```python
from build123d import *

# Parameters (mm, degrees)
F1_DEPTH = 20
F2_R     = 18
F3_DEPTH = 30
F6_D     = 10
F7_D     = 14
F7_DEPTH = 31
F7_TIP   = 4.2060243332


with BuildPart() as f1:
    # F0 (on Front) → F1 (new body)
    with BuildSketch(Plane.XZ):
        with BuildLine():
            Line((39.2857142857, 9.0350790291), (10.7142857143, 22.5876975726))
            ThreePointArc((10.7142857143, 22.5876975726), (0, 25), (-10.7142857143, 22.5876975726))
            Line((-10.7142857143, 22.5876975726), (-39.2857142857, 9.0350790291))
            ThreePointArc((-39.2857142857, 9.0350790291), (-45, 0), (-39.2857142857, -9.0350790291))
            Line((-39.2857142857, -9.0350790291), (-10.7142857143, -22.5876975726))
            ThreePointArc((-10.7142857143, -22.5876975726), (0, -25), (10.7142857143, -22.5876975726))
            Line((10.7142857143, -22.5876975726), (39.2857142857, -9.0350790291))
            ThreePointArc((39.2857142857, -9.0350790291), (45, 0), (39.2857142857, 9.0350790291))
        make_face()
    extrude(amount=F1_DEPTH)

    # F2 (on face) → F3 (join)
    with BuildSketch(Plane.XZ.offset(20)):
        Circle(F2_R)
    extrude(amount=F3_DEPTH)

    # F6 (through all)
    with Locations(Plane.XZ.offset(20)):
        with Locations((35, 0), (-35, 0)):
            Hole(F6_D / 2)

    # F7
    with Locations(Plane.XZ.offset(50)):
        with Locations((0, 0)):
            Hole(F7_D / 2, depth=F7_DEPTH)
            with Locations((0, 0, -(F7_DEPTH + F7_TIP / 2))):  # 118° drill point
                Cone(0, F7_D / 2, F7_TIP, mode=Mode.SUBTRACT)


solid = f1.part
```
The listing builds one solid part. Answer for the finished solid, in the listing's coordinates (mm). A direction names the side the tool comes from. Give positions to 0.01 mm unless a question says otherwise; leave off trailing zeros. Loops run counter-clockwise (first coordinate to the right, second up) from the corner with the lowest first, then second, coordinate; pieces in that order, holes last. Notation, with made-up numbers: (75.5, 22.25) - (105.5, 22.25) arc R29 ccw to (105.5, 51.25) - close; hole circle Ø8 at (88.5, 15). An arc over 180 degrees is marked (long way). Return JSON: item names as keys, results as strings. Group by question number.
1. Find section A-A (y = -3.5). Write down the section's boundary in (x, z), then the cut area to 3 significant figures.
2. Given pin 1 Ø11 at (x, z) = (0, 0) entering from -Y; pin 2 Ø4 at (x, z) = (-31.5, 16) entering from -Y; pin 3 Ø3 at (x, y) = (-1.5, -29) entering from +Z; pin 4 Ø1 at (y, z) = (-8, 19) entering from +X, each flat-ended and moving along its own axis, determine where each tip first touches the part or whether it passes through.
3. Find section C-C (z = 12). Write down the section's boundary in (x, y).
4. Find section B-B (x = -34). Write down the section's boundary in (y, z), then the cut area to 3 significant figures.
5. Determine the mould class of faces 1 (the conical face through (-0.264, -15.524, -1.187)), 2 (the cylindrical face through (40, -10, 0)), 3 (the cylindrical face through (-45, -10, 0)), 4 (the flat face through (24.8, -9.86, -15.906)) for opening direction Z: pulls with the +Z half, pulls with the -Z half, needs draft (parallel to the pull), parting line crosses it, or undercut.
6. Which of the six approach directions +Z, -Z, +X, -X, +Y, -Y give full straight-line access (tool end or side, diameter ignored) to faces 5 (the cylindrical face through (-6.466, -34.283, -2.681)), 6 (the cylindrical face through (0, -10, -25))?
7. Find section D-D (x = 35). Write down the section's boundary in (y, z).
8. Straight lines are drawn through the part: line 1 (Z direction, x = 0, y = -30); line 2 (Z direction, x = 35, y = -10.25); line 3 (Y direction, x = -25.5, z = -10). For each, find the intervals that lie inside material, in ascending order. Write a range as [from, to].
Verdict:
{
 "1": {"outline": "(-39.29, -9.04) - (-10.71, -22.59) arc R25 ccw to (10.71, -22.59) - (39.29, -9.04) arc R10 ccw to (39.29, 9.04) - (10.71, 22.59) arc R25 ccw to (-10.71, 22.59) - (-39.29, 9.04) arc R10 ccw to start; hole circle Ø10 at (-35, 0); hole circle Ø10 at (35, 0)", "area": "2,840 mm^2"},
 "2": {"pin 1": "stops at y = -18.1", "pin 2": "passes through", "pin 3": "stops at z = 18", "pin 4": "stops at x = 19.33"},
 "3": {"outline": "(-33.04, -20) - (-13.42, -20) - (-13.42, -50) - (13.42, -50) - (13.42, -20) - (33.04, -20) - (33.04, 0) - (-33.04, 0) - close"},
 "4": {"outline": "(-20, -11.54) - (0, -11.54) - (0, -4.9) - (-20, -4.9) - close; (-20, 4.9) - (0, 4.9) - (0, 11.54) - (-20, 11.54) - close", "area": "266 mm^2"},
 "5": {"face 1": "undercut", "face 2": "undercut", "face 3": "parting line crosses it", "face 4": "pulls with the -Z half"},
 "6": {"face 5": "-Y", "face 6": "-Z, +Y, -Y"},
 "7": {"outline": "(-20, -11.07) - (0, -11.07) - (0, -5) - (-20, -5) - close; (-20, 5) - (0, 5) - (0, 11.07) - (-20, 11.07) - close"},
 "8": {"line 1": "z = [-18, -7], [7, 18]", "line 2": "z = [-11.07, -5], [5, 11.07]", "line 3": "y = [-20, 0]"}
}
